```python
from build123d import *

# Parameters (mm, degrees)
SKETCH021_W     = 16
SKETCH021_H     = 16
PAD012_DEPTH    = 28.8
POCKET009_DEPTH = 16
PAD139_DEPTH    = 16
SKETCH192_W     = 16
SKETCH192_H     = 2
POCKET074_DEPTH = 30


with BuildPart() as part:
    # Sketch021 (on Face60 of Binder008) → Pad012 (new body)
    with BuildSketch(Plane.XY.offset(-28.8)):
        with Locations((-8, 64)):
            Rectangle(SKETCH021_W, SKETCH021_H)
    extrude(amount=PAD012_DEPTH)

    # Sketch022 (on Face3 of Pad012) → Pocket009 (cut)
    with BuildSketch(Plane.XZ.offset(-56)):
        Polygon((-16, -9.6), (0, 0), (-16, 0), align=None)
    extrude(amount=-POCKET009_DEPTH, mode=Mode.SUBTRACT)

    # Sketch139 (on Face6 of Pocket009) → Pad139 (join)
    with BuildSketch(Plane.XZ.offset(-56)):
        Polygon((0, 0), (-3.2, 0), (-16, -7.68), (-16, -10.88), (-3.2, -3.2), (0, -3.2), align=None)
    extrude(amount=-PAD139_DEPTH)

    # Sketch192 (on Face1 of Pad139) → Pocket074 (cut)
    with BuildSketch(Plane(origin=(0, 0, -28.8), x_dir=(1, 0, 0), z_dir=(0, 0, -1))):
        with Locations((-8, -57)):
            Rectangle(SKETCH192_W, SKETCH192_H)
        with Locations((-8, -71)):
            Rectangle(SKETCH192_W, SKETCH192_H)
    extrude(amount=-POCKET074_DEPTH, mode=Mode.SUBTRACT)


solid = part.part
```
Source: CAD feature listing. Evaluate the final solid. Frame: model axes, mm. Give positions to 0.01 mm unless a question says otherwise; leave off trailing zeros. Loops run counter-clockwise (first coordinate to the right, second up) from the corner with the lowest first, then second, coordinate; pieces in that order, holes last. Notation, with made-up numbers: (-16, -14) -> (13, -14) arc R30 ccw to (13, 19) -> close; hole circle Ø1 at (52, 85.5). An arc over 180 degrees is marked (long way). Use a Markdown table: item, result. Add a question column.
(1) Section query B-B (x = -10.5). Output: boundary loops of the cut face in (y, z).
(2) First-contact query: pin 1 Ø1 at (x, y) = (-5.5, 63) entering from +Z; pin 2 Ø3 at (y, z) = (64.5, -4.5) entering from -X. Flat tips, straight axial feed; report the tip coordinate or a pass-through.
(3) Section query A-A (y = 65). Output: boundary loops of the cut face in (x, z).
(4) Ray query, line 1 (Z direction, x = -6.25, y = 65.75); line 2 (Z direction, x = -5.5, y = 65.5). Return the intervals inside material, ascending.
(5) Section query C-C (x = -13.75). Output: boundary loops of the cut face in (y, z).
Checked values:
| question | item | result |
|---|---|---|
| 1 | outline | (58, -28.8) -> (70, -28.8) -> (70, -4.38) -> (58, -4.38) -> close |
| 2 | pin 1 | z = -1.08 |
| 2 | pin 2 | x = -13.2 |
| 3 | outline | (-16, -28.8) -> (0, -28.8) -> (0, 0) -> (-3.2, 0) -> (-16, -7.68) -> close |
| 4 | line 1 | -28.8 to -1.83 |
| 4 | line 2 | -28.8 to -1.38 |
| 5 | outline | (58, -28.8) -> (70, -28.8) -> (70, -6.33) -> (58, -6.33) -> close |
